Could you check a few things on this model? Use its own coordinates, in mm. A direction names the side the tool comes from. Coordinates: 2 decimals unless noted, no trailing zeros. Order: outer loops, then holes, each group sorted by start corner. A loop starts at its lowest first (then second) coordinate and runs counter-clockwise, first axis right, second up. Notation, with made-up numbers: (67.25, 30) -> (112.25, 30) arc R23 cw to (112.25, 51) -> close; hole circle Ø5 at (36.25, 59.25). An arc over 180 degrees is marked (long way). Put each result on its own line as item: value. Start each with the question number.
Q1. If we section it at D-D (z = 65.5): Count the separate pieces of the cut face and the enclosed holes in it, and give its area (3 significant figures).
Q2. If we section it at A-A (y = -22): Please give me the cut outline in (x, z).
Q3. Will these pins go through, and if not, where does the flat tip stop? pin 1 (10 mm diameter, centred on x = -29, z = 45.5, fed in from -Y); pin 2 (12 mm diameter, centred on y = -11.5, z = 57, fed in from -X); pin 3 (16.5 mm diameter, centred on y = -22, z = 43.5, fed in from -X).
Q4. Please list where these lines run through material, in increasing order: line 1 along Y through (x, z) = (-2.3, 15); line 2 along X through (y, z) = (-27.5, 28); line 3 along X through (y, z) = (-6, 15).
Q5. If we section it at C-C (x = -54.5): Please give me the cut outline in (y, z), and give its area (3 significant figures).
Q6. For faces 5 (the face through (-130, -10.992, 23)), 6 (the face through (-134.2, -13.4, 25)), 7 (the face through (-110.71, -16.73, 67.43)), which set-ups out of +Z, -Z, +X, -X, +Y, -Y let a thin tool reach every point of the face, with its end or its side?
Q7. If we section it at B-B (z = 40): Please give me the cut outline in (x, y), and give its area (3 significant figures).
Q8. We'd pull the mould along X, two halves only. Please class faces 1 (the face through (0, -6, 41)), 2 (the face through (-130, -15.992, 23)), 3 (the face through (-112.364, 4.875, 70.082)), 4 (the face through (-62, -33, 25)): +X half, -X half, draft (parallel to the pull), parting line (faces both ways), or undercut.
from build123d import *

# Parameters (mm, degrees)
ESTRUSIONE_ESTRUSIONE1_DEPTH = 5
ESTRUSIONE_SOTTILE1_START    = -33
ESTRUSIONE_SOTTILE1_DEPTH    = 33
RACCORDO1_R                  = 100
SMUSSO1_SIZE                 = 2
TAGLIO_ESTRUSIONE1_DEPTH     = 10
SCHIZZO3_R                   = 2.5
TAGLIO_ESTRUSIONE2_DEPTH     = 10
SCHIZZO3_4_R                 = 6
TAGLIO_ESTRUSIONE3_DEPTH     = 161


with BuildPart() as part:
    # Schizzo1 → Estrusione-Estrusione1 (new body)
    with BuildSketch(Plane(origin=(0, 0, 0), x_dir=(1, 0, 0), z_dir=(0, 1, 0))):
        with BuildLine():
            Line((0, -80), (0, 0))
            Line((0, 0), (-22.105704403, 0))
            Line((-22.105704403, 0), (-77.105704403, -28.023899722))
            ThreePointArc((-77.105704403, -28.023899722), (-84.735779344, -28.624399643), (-90.555674642, -23.653739478))
            Line((-90.555674642, -23.653739478), (-100.121590311, -4.879572892))
            Line((-100.121590311, -4.879572892), (-144.67191652, -27.579097879))
            Line((-144.67191652, -27.579097879), (-133.263448287, -49.969477486))
            ThreePointArc((-133.263448287, -49.969477486), (-112.995510516, -71.895209039), (-84.258089456, -80))
            Line((-84.258089456, -80), (0, -80))
        make_face()
    extrude(amount=ESTRUSIONE_ESTRUSIONE1_DEPTH)

    # Schizzo1<3> → Estrusione-Sottile1 (add)
    with BuildSketch(Plane(origin=(0, 0, 0), x_dir=(1, 0, 0), z_dir=(0, 1, 0)).offset(ESTRUSIONE_SOTTILE1_START)):
        with BuildLine():
            Line((-90.555674642, -23.653739478), (-100.121590311, -4.879572892))
            Line((-100.121590311, -4.879572892), (-144.67191652, -27.579097879))
            Line((-144.67191652, -27.579097879), (-133.263448287, -49.969477486))
            ThreePointArc((-133.263448287, -49.969477486), (-112.995510516, -71.895209039), (-84.258089456, -80))
            Line((-84.258089456, -80), (0, -80))
            Line((0, -80), (0, 0))
            Line((0, 0), (-22.105704403, 0))
            Line((-22.105704403, 0), (-77.105704403, -28.023899722))
            ThreePointArc((-77.105704403, -28.023899722), (-84.735779344, -28.624399643), (-90.555674642, -23.653739478))
        make_face()
        with BuildLine():
            Line((-95.010707263, -25.923691976), (-102.306670433, -11.604558011))
            Line((-102.306670433, -11.604558011), (-137.946931401, -29.764178001))
            Line((-137.946931401, -29.764178001), (-128.808415666, -47.699524987))
            ThreePointArc((-128.808415666, -47.699524987), (-110.383017692, -67.632008218), (-84.258089456, -75))
            Line((-84.258089456, -75), (-5, -75))
            Line((-5, -75), (-5, -5))
            Line((-5, -5), (-20.905310607, -5))
            Line((-20.905310607, -5), (-74.835751904, -32.478932343))
            ThreePointArc((-74.835751904, -32.478932343), (-86.280864316, -33.379682225), (-95.010707263, -25.923691976))
        make_face(mode=Mode.SUBTRACT)
    extrude(amount=ESTRUSIONE_SOTTILE1_DEPTH)

    # Raccordo1
    # the kernel refuses this fillet: 100 mm, written as the material it takes off along each edge
    with BuildSketch(Plane(origin=(-22.105704403, -92.916153629, 0), x_dir=(-0.8910065241883712, 0, 0.4539904997395403), z_dir=(0, 1, 0))) as raccordo1_piece_1:
        with BuildLine():
            CenterArc((23.966461452, 100), RACCORDO1_R, 244.111076085, 25.888923915)
            Line((-19.696326845, 10.035779789), (-20.569582611, 8.236495385))
            ThreePointArc((-20.569582611, 8.236495385), (-10.756144422, 3.235876846), (-0.907980999, -1.782013048))
            Line((-0.907980999, -1.782013048), (0, -2))
            Line((0, -2), (23.966461452, -2))
            Line((23.966461452, -2), (23.966461452, 0))
        make_face()
    extrude(amount=157.832307258, mode=Mode.SUBTRACT)

    # Smusso1
    smusso1_edges = [part.edges().sort_by_distance(p)[0] for p in [
        (-84.735779344, 5, 28.624399643),
        (-95.338632476, 5, 14.266656185),
        (-138.967682403, 5, 38.774287682),
        (-112.995510516, 5, 71.895209039),
        (-42.129044728, 5, 80),
        (-60.28284116, 5, 19.452222767),
        (-22.347158994, 5, 2.975121197),
    ]]
    chamfer(smusso1_edges, length=SMUSSO1_SIZE)

    # Schizzo2 → Taglio-Estrusione1 (cut)
    with BuildSketch(Plane(origin=(-18.661969348, 0, -36.626177095), x_dir=(-0.8910065241883686, 0, 0.4539904997395456), z_dir=(-0.4539904997395456, 0, -0.8910065241883686))):
        with BuildLine():
            Line((104.424269915, -10.991811), (108.424269915, -10.991811))
            ThreePointArc((108.424269915, -10.991811), (110.924269915, -13.491811), (108.424269915, -15.991811))
            Line((108.424269915, -15.991811), (104.424269915, -15.991811))
            ThreePointArc((104.424269915, -15.991811), (101.924269915, -13.491811), (104.424269915, -10.991811))
        make_face()
        with BuildLine():
            Line((124.424269915, -10.991811), (128.424269915, -10.991811))
            ThreePointArc((128.424269915, -10.991811), (130.924269915, -13.491811), (128.424269915, -15.991811))
            Line((128.424269915, -15.991811), (124.424269915, -15.991811))
            ThreePointArc((124.424269915, -15.991811), (121.924269915, -13.491811), (124.424269915, -10.991811))
        make_face()
    extrude(amount=-TAGLIO_ESTRUSIONE1_DEPTH, mode=Mode.SUBTRACT)

    # Schizzo3 → Taglio-Estrusione2 (cut)
    with BuildSketch(Plane(origin=(0, 0, 0), x_dir=(0, 0, -1), z_dir=(1, 0, 0))):
        with Locations((-65, -26)):
            Circle(SCHIZZO3_R)
        with Locations((-65, -7)):
            Circle(SCHIZZO3_R)
        with Locations((-15, -7)):
            Circle(SCHIZZO3_R)
        with Locations((-15, -26)):
            Circle(SCHIZZO3_R)
    extrude(amount=-TAGLIO_ESTRUSIONE2_DEPTH, mode=Mode.SUBTRACT)

    # Schizzo3<4> → Taglio-Estrusione3 (cut)
    with BuildSketch(Plane(origin=(0, 0, 0), x_dir=(0, 0, -1), z_dir=(1, 0, 0))):
        with Locations((-40, -14)):
            Circle(SCHIZZO3_4_R)
    extrude(amount=-TAGLIO_ESTRUSIONE3_DEPTH, mode=Mode.SUBTRACT)


solid = part.part
The answers:
1. separate pieces: 3
1. enclosed holes: 0
1. area: 981 mm^2
2. outline: (-144.67, 27.58) -> (-100.12, 4.88) -> (-90.56, 23.65) arc R10 cw to (-77.11, 28.02) -> (-43.46, 10.88) arc R100 ccw to (0, 0) -> (0, 80) -> (-84.26, 80) arc R55 ccw to (-133.26, 49.97) -> close; hole (-137.95, 29.76) -> (-102.31, 11.6) -> (-95.01, 25.92) arc R15 cw to (-74.84, 32.48) -> (-20.91, 5) -> (-5, 5) -> (-5, 75) -> (-84.26, 75) arc R50 ccw to (-128.81, 47.7) -> close
3. pin 1: y = 0
3. pin 2: x = -132.72
3. pin 3: x = -140.76
4. line 1: -33 to -28.5, -23.5 to -9.5, -4.5 to 5
4. line 2: -144.46 to -134.48, -93.73 to -86.23, -77.06 to -66.05, -5 to 0
4. line 3: -119.98 to -108.97, -100.58 to -94.96, -51.54 to -40.53
5. outline: (-33, 16.51) -> (3, 16.51) -> (5, 18.75) -> (5, 78) -> (3, 80) -> (-33, 80) -> (-33, 75) -> (0, 75) -> (0, 22.12) -> (-33, 22.12) -> close
5. area: 663 mm^2
6. face 5: none
6. face 6: -Z
6. face 7: -Y
7. outline: (-138.34, -33) -> (-132.73, -33) -> (-132.73, -20) -> (-138.34, -20) -> close; (-138.34, -8) -> (-132.73, -8) -> (-132.73, 0) -> (-5, 0) -> (-5, -8) -> (0, -8) -> (0, 5) -> (-136.1, 5) -> (-138.34, 3) -> close; (-5, -33) -> (0, -33) -> (0, -20) -> (-5, -20) -> close
7. area: 912 mm^2
8. face 1: +X half
8. face 2: undercut
8. face 3: -X half
8. face 4: draft
